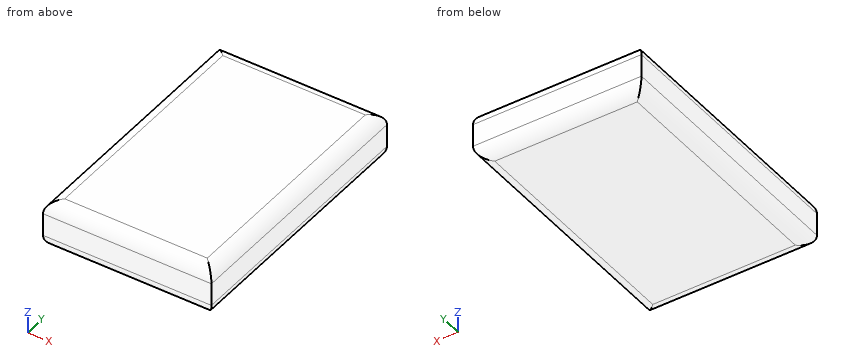
```python
from build123d import *

# Parameters (mm, degrees)
SKETCH1_W           = 33.02
SKETCH1_H           = 50.8
BOSS_EXTRUDE1_DEPTH = 9.525
FILLET1_R           = 2.54


with BuildPart() as part:
    # Sketch1 → Boss-Extrude1 (new body)
    with BuildSketch(Plane.XY):
        Rectangle(SKETCH1_W, SKETCH1_H)
    extrude(amount=BOSS_EXTRUDE1_DEPTH)

    # Fillet1
    fillet1_edges = [part.edges().sort_by_distance(p)[0] for p in [
        (16.51, 0, 9.525),
        (0, 25.4, 9.525),
        (-16.51, 0, 9.525),
        (0, 25.4, 0),
        (16.51, 0, 0),
        (0, -25.4, 0),
        (-16.51, 0, 0),
        (0, -25.4, 9.525),
    ]]
    fillet(fillet1_edges, radius=FILLET1_R)


solid = part.part
```
The model under review builds one solid part; all positions refer to its coordinate system, in mm. Round coordinates to 2 decimals unless told otherwise and drop trailing zeros. Write each loop counter-clockwise with the first axis right and the second up, starting at its lowest first coordinate (ties: lowest second). Pieces come first, ordered by that corner, then holes.
(1) We need section A-A on y = -19. Give the boundary of the cut face in (x, z) (3 decimals).
(2) Insertion check: pin 1 (5 mm diameter, centred on x = -3.5, z = 2, fed in from +Y). The pin has a flat end and moves straight along its axis. Give the tip position at first contact, or say it passes through.
(3) Wall thickness on L1, parallel to X at y = -22.5, z = 1.25; L2, parallel to Y at x = -12.5, z = 2.25; L3, parallel to Y at x = -13, z = 2: over which ranges is each line inside the solid? List them lowest first.
(4) We need section B-B on z = 8. Give the boundary of the cut face in (x, y).
(5) We need section C-C on z = 0.5. Give the boundary of the cut face in (x, y), and give its area (3 significant figures).
Findings below:
1. outline: (-16.51, 2.54) arc R2.54 ccw to (-13.97, 0) - (13.97, 0) arc R2.54 ccw to (16.51, 2.54) - (16.51, 6.985) arc R2.54 ccw to (13.97, 9.525) - (-13.97, 9.525) arc R2.54 ccw to (-16.51, 6.985) - close
2. pin 1: stops at y = 25.4
3. L1: x = -16.16 to 16.16
3. L2: y = -25.38 to 25.38
3. L3: y = -25.34 to 25.34
4. outline: (-16.3, -25.19) - (16.3, -25.19) - (16.3, 25.19) - (-16.3, 25.19) - close
5. outline: (-15.48, -24.37) - (15.48, -24.37) - (15.48, 24.37) - (-15.48, 24.37) - close
5. area: 1,510 mm2
